Build history of the part. All positions in model axes, mm. Face numbers are marked on the shaded views. Round coordinates to 2 decimals unless told otherwise and drop trailing zeros. Write each loop counter-clockwise with the first axis right and the second up, starting at its lowest first coordinate (ties: lowest second). Pieces come first, ordered by that corner, then holes. Notation, with made-up numbers: (16, -39.75) -> (59, -39.75) arc R17 ccw to (59, -26.75) -> close; hole circle Ø5 at (20.5, 35). An arc over 180 degrees is marked (long way). Return JSON: item names as keys, results as strings.
from build123d import *

# Parameters (mm, degrees)
F0_R     = 4
F1_DEPTH = 8
F4_SIZE  = 0.5


# Not quite as in the source:
# - a feature of the source that left no trace in its solid (it failed there, or was rolled back) is left out


with BuildPart() as f1:
    # F0 (on Top) → F1 (new body)
    with BuildSketch(Plane.XY):
        Polygon((4.9074772881, -8.5), (9.8149545762, 0), (4.9074772881, 8.5), (-4.9074772881, 8.5), (-9.8149545762, 0), (-4.9074772881, -8.5), align=None)
        Circle(F0_R, mode=Mode.SUBTRACT)
    extrude(amount=F1_DEPTH)

    # F2 (on Front) → F3 (revolve, cut)
    with BuildSketch(Plane.XZ):
        Polygon((12.4901464933, 8), (8.25, 8), (12.4901464933, 5.5519502807), align=None)
        Polygon((12.4901464933, 2.4480497193), (8.25, 0), (12.4901464933, 0), align=None)
    revolve(axis=Axis((0, 0, 3.4472336993), (0, 0, -1)), mode=Mode.SUBTRACT)

    # F4
    f4_edges = [f1.edges().sort_by_distance(p)[0] for p in [
        (-4, 0, 8),
        (-4, 0, 0),
    ]]
    chamfer(f4_edges, length=F4_SIZE)


solid = f1.part
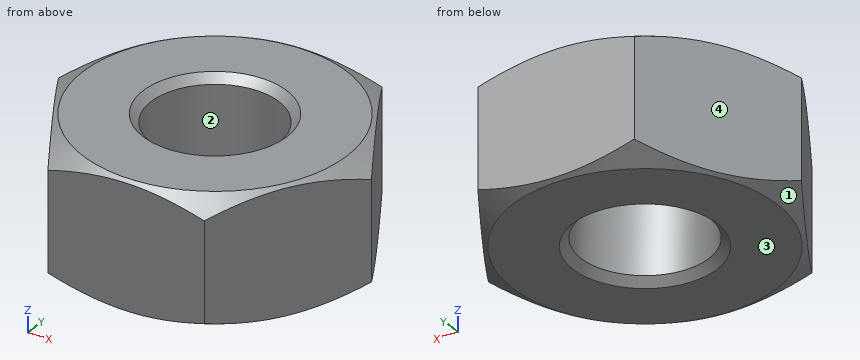
Q1. Pin check, flat tip, straight feed: pin 1 Ø1.5 at (x, y) = (-2, -0.5) entering from +Z. Stop position of the tip, or through.
Verdict:
{"pin 1": "passes through"}
Q2. Saw through at A-A on x = 0. List the corners of the cut face in (y, z), then the cut area to 3 significant figures.
Verdict:
{"outline": "(-8.5, 0.14) -> (-8.25, 0) -> (-4.5, 0) -> (-4, 0.5) -> (-4, 7.5) -> (-4.5, 8) -> (-8.25, 8) -> (-8.5, 7.86) -> close; (4, 0.5) -> (4.5, 0) -> (8.25, 0) -> (8.5, 0.14) -> (8.5, 7.86) -> (8.25, 8) -> (4.5, 8) -> (4, 7.5) -> close", "area": "71.4 mm²"}
Q3. Saw through at B-B on z = 4.25. List the corners of the cut face in (x, y).
Verdict:
{"outline": "(-9.81, 0) -> (-4.91, -8.5) -> (4.91, -8.5) -> (9.81, 0) -> (4.91, 8.5) -> (-4.91, 8.5) -> close; hole circle Ø8 at (0, 0)"}
Q4. Wall check: L1, parallel to Y at x = 0, z = 3.5; L2, parallel to X at y = -1.75, z = 3.25; L3, parallel to Y at x = -3.5, z = 7. Give the ranges that are in metal, low to high.
Verdict:
{"L1": "y = -8.5 to -4, 4 to 8.5", "L2": "x = -8.8 to -3.6, 3.6 to 8.8", "L3": "y = -8.5 to -1.94, 1.94 to 8.5"}
Q5. Two-plate mould, pull along X, no slides. Class the marked faces 1, 2, 3 and 4: +X half, -X half, draft (parallel to the pull), parting line (faces both ways), or undercut.
Verdict:
{"face 1": "parting line", "face 2": "undercut", "face 3": "draft", "face 4": "-X half"}
